Input: part model. Units: mm. Frame: model coordinates. Give positions to 0.01 mm unless a question says otherwise; leave off trailing zeros. Order: outer loops, then holes, each group sorted by start corner. A loop starts at its lowest first (then second) coordinate and runs counter-clockwise, first axis right, second up. Notation, with made-up numbers: M 55.25,-21.75 L 86.25,-21.75 A21 cw 86.25,14.25 Z; hole C 30.25,10.25 d1. An arc over 180 degrees is marked long. Use a Markdown table: item, result.
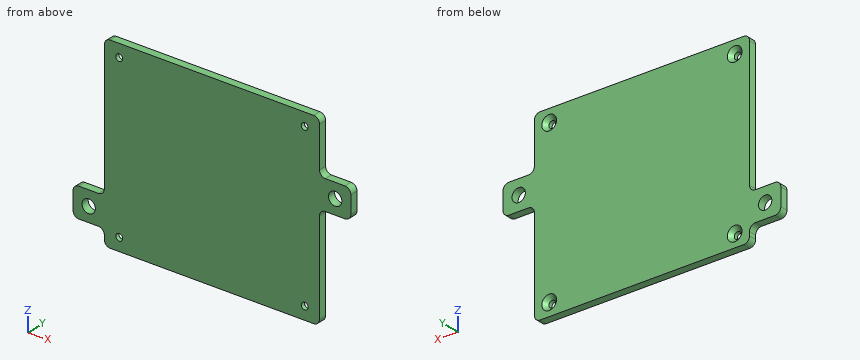
Autodesk Fusion 360 part; units mm, degrees
sketch "Sketch1" plane through (0, 0, 0) normal (0, 1, 0) x (1, 0, 0)
  line L0 (47.35, 40.9) -> (-47.35, 40.9) construction
  line L1 (-47.35, 40.9) -> (-47.35, -40.9) construction
  line L2 (-47.35, -40.9) -> (47.35, -40.9) construction
  line L3 (47.35, -40.9) -> (47.35, 40.9) construction
  line L4 (47.35, 40.9) -> (-47.35, -40.9) construction
  line L5 (-47.35, 40.9) -> (47.35, -40.9) construction
  line L6 (54.9177, 47.4368) -> (-54.9177, 47.4368)
  line L7 (-54.9177, 47.4368) -> (-54.9177, -47.4368)
  line L8 (-54.9177, -47.4368) -> (54.9177, -47.4368)
  line L9 (54.9177, -47.4368) -> (54.9177, 47.4368)
  line L10 (54.9177, 47.4368) -> (-54.9177, -47.4368) construction
  line L11 (-54.9177, 47.4368) -> (54.9177, -47.4368) construction
  circle A0 centre (47.35, 40.9) radius 1.75
  line L12 (0, 0) -> (0, 35) construction
  line L13 (0, 0) -> (-41.0628, 0) construction
  circle A1 centre (-47.35, 40.9) radius 1.75
  circle A2 centre (47.35, -40.9) radius 1.75
  circle A3 centre (-47.35, -40.9) radius 1.75
  line L14 (-54.9177, 39.4) -> (-70.9177, 39.4)
  line L15 (-70.9177, 39.4) -> (-70.9177, 24.4)
  line L16 (-70.9177, 24.4) -> (-54.9177, 24.4)
  line L17 (-54.9177, 24.4) -> (-54.9177, 39.4)
  line L18 (54.9177, -5.6) -> (70.9177, -5.6)
  line L19 (70.9177, -5.6) -> (70.9177, -20.6)
  line L20 (70.9177, -20.6) -> (54.9177, -20.6)
  line L21 (54.9177, -20.6) -> (54.9177, -5.6)
  line L22 (81.8257, 31.9) -> (62.2169, 31.9) construction
  line L23 (80.3912, -13.1) -> (59.348, -13.1) construction
  circle A4 centre (-62.9177, 31.9) radius 3.4
  circle A5 centre (62.9177, -13.1) radius 3.4
  dimension "d1" = 3.5
  dimension "d2" = 81.8
  dimension "d3" = 94.7
  dimension "d4" = 10
  dimension "d5" = 16
  dimension "d6" = 15
  dimension "d7" = 15
  dimension "d9" = 16
  dimension "d10" = 45
  dimension "d11" = 9
  dimension "d12" = 6.8
  dimension "d13" = 6.8
  dimension "d14" = 8
  dimension "d15" = 8
extrude "Extrude1" add sketch "Sketch1" along normal blind 4
fillet "Fillet1" radius 3 12 edges at (-70.9177, 2, -24.4) (-70.9177, 2, -39.4) (-54.9177, 2, -39.4) (-54.9177, 2, -47.4368) (-54.9177, 2, 47.4368) (-54.9177, 2, -24.4) (54.9177, 2, 47.4368) (54.9177, 2, 20.6) (70.9177, 2, 20.6) (70.9177, 2, 5.6) (54.9177, 2, 5.6) (54.9177, 2, -47.4368)
chamfer "Chamfer1" distance 2 angle 45 4 edges at (45.7184, 4, 40.2672) (-48.9816, 4, 40.2672) (-48.9816, 4, -41.5328) (45.7184, 4, -41.5328)
1) Cut plane C-C on x = 47.35. Return loops of the section in (y, z), and give its area (3 significant figures).
Response values:
| item | result |
|---|---|
| outline | M 0,-47.44 L 4,-47.44 L 4,-44.65 L 2,-42.65 L 0,-42.65 Z; M 0,-39.15 L 2,-39.15 L 4,-37.15 L 4,37.15 L 2,39.15 L 0,39.15 Z; M 0,42.65 L 2,42.65 L 4,44.65 L 4,47.44 L 0,47.44 Z |
| area | 343 mm² |
2) First-contact query: pin 1 Ø5.5 at (x, z) = (-47.35, -40.9) entering from +Y; pin 2 Ø0.6 at (y, z) = (2.5, -44) entering from -X; pin 3 Ø4 at (x, z) = (-47.35, 40.9) entering from -Y. Flat tips, straight axial feed; report the tip coordinate or a pass-through.
Response values:
| item | result |
|---|---|
| pin 1 | stops at y = 3 |
| pin 2 | stops at x = -54.92 |
| pin 3 | stops at y = 0 |
3) Cut plane B-B on y = 1. State how many separate pieces and enclosed holes the cut face has, and give its area (3 significant figures).
Response values:
| item | result |
|---|---|
| separate pieces | 1 |
| enclosed holes | 6 |
| area | 10,800 mm² |
4) Material intervals for line 1 (X direction, y = 1.5, z = 40.9); line 2 (Z direction, x = 47.35, y = 0.8); line 3 (X direction, y = 1.8, z = -31.9), sorted ascending. Write a range as from..to.
Response values:
| item | result |
|---|---|
| line 1 | x = -54.92..-49.1, -45.6..45.6, 49.1..54.92 |
| line 2 | z = -47.44..-42.65, -39.15..39.15, 42.65..47.44 |
| line 3 | x = -70.92..-66.32, -59.52..54.92 |
5) Cut plane A-A on z = 13.1. Return loops of the section in (x, y).
Response values:
| item | result |
|---|---|
| outline | M -54.92,0 L 59.52,0 L 59.52,4 L -54.92,4 Z; M 66.32,0 L 70.92,0 L 70.92,4 L 66.32,4 Z |
6) Cut plane D-D on z = 40.9. Return loops of the section in (x, y), and give its area (3 significant figures).
Response values:
| item | result |
|---|---|
| outline | M -54.92,0 L -49.1,0 L -49.1,2 L -51.1,4 L -54.92,4 Z; M -45.6,0 L 45.6,0 L 45.6,2 L 43.6,4 L -43.6,4 L -45.6,2 Z; M 49.1,0 L 54.92,0 L 54.92,4 L 51.1,4 L 49.1,2 Z |
| area | 403 mm² |
